from build123d import *

# Parameters (mm, degrees)
ESQUISSE1_W             = 86
ESQUISSE1_H             = 10
BOSS_EXTRU_1_DEPTH      = 1
ESQUISSE2_W             = 86
ESQUISSE2_H             = 1
BOSS_EXTRU_2_DEPTH      = 8
ESQUISSE3_R             = 1.25
ENL_V_MAT_EXTRU_1_DEPTH = 10
ESQUISSE4_R             = 1.25
ENL_V_MAT_EXTRU_2_DEPTH = 10
ESQUISSE5_W             = 46
ESQUISSE5_H             = 5
ENL_V_MAT_EXTRU_3_DEPTH = 10
ESQUISSE6_W             = 46
ESQUISSE6_H             = 5
ENL_V_MAT_EXTRU_4_DEPTH = 10
ESQUISSE8_R             = 2.5
ENL_V_MAT_EXTRU_5_DEPTH = 10


with BuildPart() as part:
    # Esquisse1 → Boss.-Extru.1 (new body)
    with BuildSketch(Plane(origin=(0, 0, 0), x_dir=(1, 0, 0), z_dir=(0, 1, 0))):
        with Locations((-31.256880734, 5.871559633)):
            Rectangle(ESQUISSE1_W, ESQUISSE1_H)
    extrude(amount=BOSS_EXTRU_1_DEPTH)

    # Esquisse2 → Boss.-Extru.2 (add)
    with BuildSketch(Plane(origin=(0, 1, 0), x_dir=(1, 0, 0), z_dir=(0, 1, 0))):
        with Locations((-31.256880734, 10.371559633)):
            Rectangle(ESQUISSE2_W, ESQUISSE2_H)
    extrude(amount=BOSS_EXTRU_2_DEPTH)

    # Esquisse3 → Enlèv. mat.-Extru.1 (cut)
    with BuildSketch(Plane.XY.offset(-9.871559633)):
        with Locations((8.743119266, 5)):
            Circle(ESQUISSE3_R)
        with Locations((-71.256880734, 5)):
            Circle(ESQUISSE3_R)
    extrude(amount=-ENL_V_MAT_EXTRU_1_DEPTH, mode=Mode.SUBTRACT)

    # Esquisse4 → Enlèv. mat.-Extru.2 (cut)
    with BuildSketch(Plane(origin=(0, 1, 0), x_dir=(1, 0, 0), z_dir=(0, 1, 0))):
        with Locations(Location((-61.256880734, 4.871559633, 0), (0, 0, 270))):  # turned: the seam where the file's is
            Circle(ESQUISSE4_R)
        with Locations(Location((-1.256880734, 4.871559633, 0), (0, 0, 270))):  # turned: the seam where the file's is
            Circle(ESQUISSE4_R)
    extrude(amount=-ENL_V_MAT_EXTRU_2_DEPTH, mode=Mode.SUBTRACT)

    # Esquisse5 → Enlèv. mat.-Extru.3 (cut)
    with BuildSketch(Plane(origin=(0, 1, 0), x_dir=(1, 0, 0), z_dir=(0, 1, 0))):
        with Locations((-31.256880734, 3.371559633)):
            Rectangle(ESQUISSE5_W, ESQUISSE5_H)
    extrude(amount=-ENL_V_MAT_EXTRU_3_DEPTH, mode=Mode.SUBTRACT)

    # Esquisse6 → Enlèv. mat.-Extru.4 (cut)
    with BuildSketch(Plane.XY.offset(-9.871559633)):
        with Locations((-31.256880734, 6.5)):
            Rectangle(ESQUISSE6_W, ESQUISSE6_H)
    extrude(amount=-ENL_V_MAT_EXTRU_4_DEPTH, mode=Mode.SUBTRACT)

    # Esquisse8 → Enlèv. mat.-Extru.5 (cut)
    with BuildSketch(Plane.XY.offset(-9.871559633)):
        with Locations((-46.256880734, 4)):
            Circle(ESQUISSE8_R)
    extrude(amount=-ENL_V_MAT_EXTRU_5_DEPTH, mode=Mode.SUBTRACT)


solid = part.part
Geometry check sheet. Reference: the model listing, model coordinates, mm. Give positions to 0.01 mm unless a question says otherwise; leave off trailing zeros. Loops run counter-clockwise (first coordinate to the right, second up) from the corner with the lowest first, then second, coordinate; pieces in that order, holes last. Notation, with made-up numbers: (44, 76.5) -> (66, 76.5) arc R24 cw to (66, 101.5) -> close; hole circle Ø4 at (3, 27). An arc over 180 degrees is marked (long way). Answer in a Markdown table with one row per item. Add a question column.
1) Draft check along Z on faces 1 (the face through (-31.9, 1, -6.4)), 2 (the face through (-32, 3, -9.872)), 3 (the face through (-1.2, 0.51, -6.12)), 4 (the face through (-60.018, 0.507, -5.034)). Enter one of: pulls with the +Z half, pulls with the -Z half, needs draft (parallel to the pull), parting line crosses it, or undercut.
2) Gauge pin test, flat ends, axial feed: P1, Ø0.8, axis at x = -52.5, z = -10.5, coming from the +Y side; P2, Ø3, axis at x = -1.26, z = -4.87, coming from the +Y side; P3, Ø1.1, axis at x = -21.5, y = 0.5, coming from the +Z side. Record the tip position at first contact, or that the pin passes through.
3) Cross-section at A-A on y = 5. Record the boundary of the cut face in (x, z), and give its area (3 significant figures).
4) Cross-section at B-B on x = -3.5. Record the boundary of the cut face in (y, z).
5) Material ranges on probe 1 along Z at (x, y) = (7.5, 1.75); probe 2 along Y at (x, z) = (-7, -2); probe 3 along Y at (x, z) = (-38, -10), recorded low to high. Write a range as from..to.
6) Cross-section at C-C on x = -52.5. Record the boundary of the cut face in (y, z), and give its area (3 significant figures).
Outcome:
| question | item | result |
|---|---|---|
| 1 | face 1 | needs draft |
| 1 | face 2 | pulls with the +Z half |
| 1 | face 3 | undercut |
| 1 | face 4 | undercut |
| 2 | P1 | stops at y = 4 |
| 2 | P2 | stops at y = 1 |
| 2 | P3 | stops at z = -5.87 |
| 3 | outline | (-74.26, -10.87) -> (-72.51, -10.87) -> (-72.51, -9.87) -> (-74.26, -9.87) -> close; (-70.01, -10.87) -> (-54.26, -10.87) -> (-54.26, -9.87) -> (-70.01, -9.87) -> close; (-8.26, -10.87) -> (7.49, -10.87) -> (7.49, -9.87) -> (-8.26, -9.87) -> close; (9.99, -10.87) -> (11.74, -10.87) -> (11.74, -9.87) -> (9.99, -9.87) -> close |
| 3 | area | 35.0 mm^2 |
| 4 | outline | (0, -10.87) -> (9, -10.87) -> (9, -9.87) -> (1, -9.87) -> (1, -0.87) -> (0, -0.87) -> close |
| 5 | probe 1 | z = -10.87..-9.87 |
| 5 | probe 2 | y = 0..1 |
| 5 | probe 3 | y = 0..4 |
| 6 | outline | (0, -10.87) -> (4, -10.87) -> (4, -9.87) -> (1, -9.87) -> (1, -5.87) -> (0, -5.87) -> close |
| 6 | area | 8.00 mm^2 |
